Verification items for this drawing (mm, ordinates from the low corner). A direction names the side the tool comes from. Round coordinates to 2 decimals unless told otherwise and drop trailing zeros. Write each loop counter-clockwise with the first axis right and the second up, starting at its lowest first coordinate (ties: lowest second). Pieces come first, ordered by that corner, then holes.
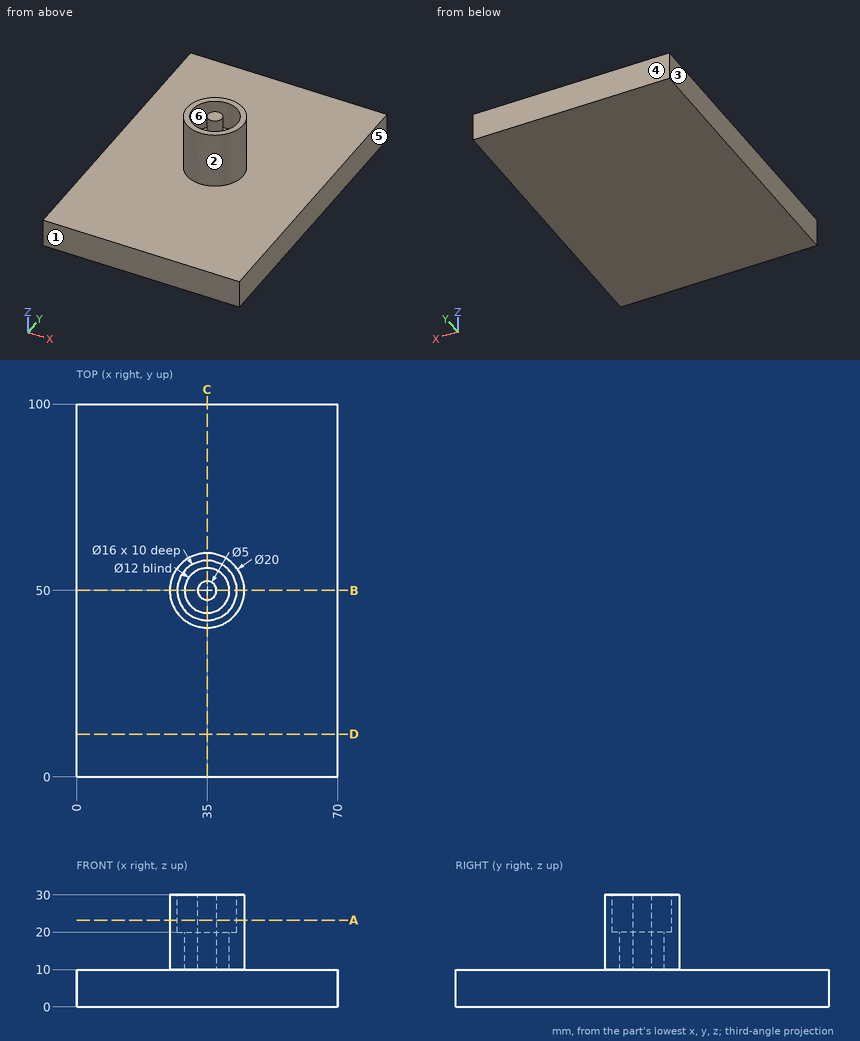
1. Release check for a two-part mould opening along X. For the marked faces 3, 4, 5 and 6 record: +X half, -X half, draft (parallel to the pull), parting line (faces both ways), or undercut.
2. Section check C-C (x = 35). Record the cut outline in (y, z), plus the area to 3 significant figures.
3. Section check A-A (z = 23.25). Record the cut outline in (x, y), plus the area to 3 significant figures.
4. Section check D-D (y = 11.5). Record the cut outline in (x, z).
5. Depth check by flat-ended pin: pin 1 Ø7 at (x, y) = (35, 50) entering from -Z; pin 2 Ø1 at (x, y) = (17, 75.5) entering from +Z. Enter the tip coordinate at first touch or a pass-through.
6. Scan lines: line 1 along Y through (x, z) = (35, 24.5); line 2 along X through (y, z) = (50, 24.25); line 3 along Y through (x, z) = (35, 15.75). Record each from-to range of solid material in increasing order.
7. Section check B-B (y = 50). Record the cut outline in (x, z), plus the area to 3 significant figures.
8. Access from +Z, -Z, +X, -X, +Y, -Y to the whole of each face (thin tool, end or side, straight path). Record for the marked faces 1 and 2.
Results below:
1. face 3: -X half
1. face 4: draft
1. face 5: +X half
1. face 6: undercut
2. outline: (0, 0) - (100, 0) - (100, 10) - (60, 10) - (60, 30) - (58, 30) - (58, 20) - (56, 20) - (56, 10) - (52.5, 10) - (52.5, 30) - (47.5, 30) - (47.5, 10) - (44, 10) - (44, 20) - (42, 20) - (42, 30) - (40, 30) - (40, 10) - (0, 10) - close
2. area: 1,220 mm2
3. outline: circle Ø20 at (35, 50); circle Ø5 at (35, 50); hole circle Ø16 at (35, 50)
3. area: 133 mm2
4. outline: (0, 0) - (70, 0) - (70, 10) - (0, 10) - close
5. pin 1: stops at z = 0
5. pin 2: stops at z = 10
6. line 1: y = 40 to 42, 47.5 to 52.5, 58 to 60
6. line 2: x = 25 to 27, 32.5 to 37.5, 43 to 45
6. line 3: y = 40 to 44, 47.5 to 52.5, 56 to 60
7. outline: (0, 0) - (70, 0) - (70, 10) - (45, 10) - (45, 30) - (43, 30) - (43, 20) - (41, 20) - (41, 10) - (37.5, 10) - (37.5, 30) - (32.5, 30) - (32.5, 10) - (29, 10) - (29, 20) - (27, 20) - (27, 30) - (25, 30) - (25, 10) - (0, 10) - close
7. area: 920 mm2
8. face 1: +Z, -Z, +X, -X, -Y
8. face 2: +Z
